from build123d import *

# Parameters (mm, degrees)
F2_R = 15


with BuildPart() as f1:
    # F0 (on Front) → F1 (revolve)
    with BuildSketch(Plane.XZ):
        Polygon((-34.2265, 0), (-30.4165, 0), (-29.077178, 2.319773), (-28.083861, 35.56), (-27.639419, 40.64), (-11.17, 85.658427), (-11.17, 120.65), (-14.98, 120.65), (-16.300187, 118.363368), (-17.018, 85.658427), (-34.2265, 38.619754), align=None)
    revolve(axis=Axis((0, 0, 84.68134), (0, 0, 1)))

    # F2
    f2_edges = [f1.edges().sort_by_distance(p)[0] for p in [
        (34.2265, 0, 38.619754),
        (17.018, 0, 85.658427),
        (11.17, 0, 85.658427),
    ]]
    fillet(f2_edges, radius=F2_R)


solid = f1.part
Work out the finished part from the listing and answer in its coordinate system (mm). A direction names the side the tool comes from. Give positions to 0.01 mm unless a question says otherwise; leave off trailing zeros. Use a Markdown table: item, result. Add a question column.
1. Find the intervals of material crossed by probe 1 along X at (y, z) = (-19, 49.5); probe 2 along Y at (x, z) = (0, 99.5); probe 3 along X at (y, z) = (0, 98.5), in increasing order.
2. Flat-ended cylindrical pins translate along their axes: pin 1 Ø4 at (y, z) = (8, 60.5) entering from +X; pin 2 Ø5 at (x, z) = (7, 55) entering from +Y; pin 3 Ø2 at (y, z) = (15.5, 24) entering from +X; pin 4 Ø13.5 at (x, y) = (0, 0) entering from +Z. Find the tip coordinate at first contact, or state that the pin passes through.
3. For faces 5 (the conical face through (-15.868, -4.997, 103.043)), 6 (the cylindrical face through (-6, -9.42, 104.71)), determine the directions among +Z, -Z, +X, -X, +Y, -Y from which every point of the face is accessible in a straight line to the end or side of a thin tool.
4. Determine the mould class of faces 1 (the conical face through (14.303, 10.967, 66.924)), 2 (the flat face through (-6, 10, 120.65)), 3 (the conical face through (3.3, 14.7, 120.5)), 4 (the conical face through (-26.395, 10.944, 19.173)) for opening direction X: released by +X, released by -X, zero draft, split by the parting line, or undercut.
Results below:
| question | item | result |
|---|---|---|
| 1 | probe 1 | x = -23.53 to -15.31, 15.31 to 23.53 |
| 1 | probe 2 | y = -16.71 to -11.17, 11.17 to 16.71 |
| 1 | probe 3 | x = -16.74 to -11.17, 11.17 to 16.74 |
| 2 | pin 1 | stops at x = 25.93 |
| 2 | pin 2 | stops at y = 28.45 |
| 2 | pin 3 | stops at x = 31 |
| 2 | pin 4 | passes through |
| 3 | face 5 | +Z |
| 3 | face 6 | +Z, -Z |
| 4 | face 1 | undercut |
| 4 | face 2 | zero draft |
| 4 | face 3 | split by the parting line |
| 4 | face 4 | undercut |
